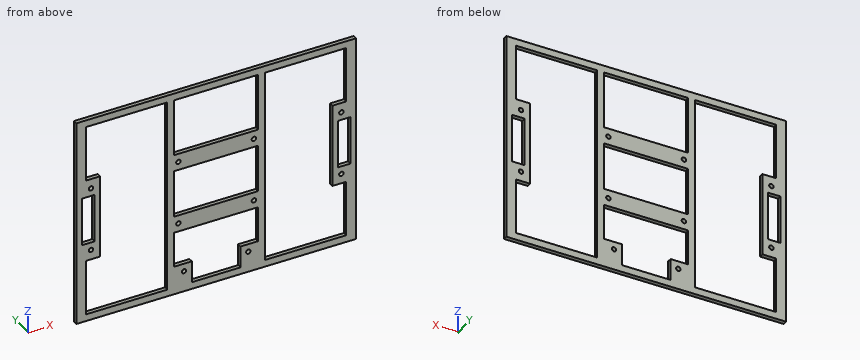
Autodesk Inventor part; units mm, degrees
ref_plane "YZ Plane" through (0, 0, 0) normal (1, 0, 0) x (0, 1, 0)
ref_plane "XZ Plane" through (0, 0, 0) normal (0, 1, 0) x (-1, 0, 0)
ref_plane "XY Plane" through (0, 0, 0) normal (0, 0, 1) x (1, 0, 0)
sketch "Skizze1" plane through (0, 0, 0) normal (0, 1, 0) x (-1, 0, 0)
  line L0 (100, -75) -> (-100, -75)
  line L1 (-100, -75) -> (-100, 75)
  line L2 (-100, 75) -> (100, 75)
  line L3 (100, 75) -> (100, -75)
  line L4 (0, -105) -> (0, 105)
  line L5 (-140, 0) -> (140, 0)
  point P0 (0, 0)
  dimension "d0" = 200
  dimension "d1" = 150
extrude "Extrusion1" add sketch "Skizze1" along normal blind 3
sketch "Skizze11" plane through (0, 3, 0) normal (0, 1, 0) x (1, 0, 0)
  circle A0 centre (27, -23) radius 1.6
  circle A1 centre (27, 23) radius 1.6
  line L0 (140, 0) -> (-140, 0)
  line L1 (100, -75) -> (100, 75)
  line L2 (100, -75) -> (100, 75)
  line L3 (0, 105) -> (0, -105)
  circle A2 centre (-27, -23) radius 1.6
  circle A3 centre (-27, 23) radius 1.6
  circle A4 centre (27, 23) radius 1.6
  circle A5 centre (-27, 23) radius 1.6
  line L4 (100, 75) -> (-100, 75)
  circle A6 centre (89.5, -23) radius 1.6
  circle A7 centre (89.5, 23) radius 1.6
  circle A8 centre (-89.5, -23) radius 1.6
  circle A9 centre (-89.5, 23) radius 1.6
  line L5 (-100, 75) -> (-100, -75)
  point P0 (0, 0)
  dimension "d50" = 3.2
  dimension "d51" = 3.2
  dimension "d52" = 23
  dimension "d53" = 23
  dimension "d54" = 73
  dimension "d55" = 73
  dimension "d62" = 3.2
  dimension "d63" = 3.2
  dimension "d64" = 27
  dimension "d65" = 27
  dimension "d66" = 52
  dimension "d67" = 52
  dimension "d70" = 3.2
  dimension "d71" = 3.2
  dimension "d72" = 23
  dimension "d73" = 23
  dimension "d74" = 10.5
  dimension "d75" = 10.5
  dimension "d76" = 3.2
  dimension "d77" = 3.2
  dimension "d78" = 10.5
  dimension "d79" = 10.5
  dimension "d80" = 23
  dimension "d81" = 23
extrude "Extrusion12" cut sketch "Skizze11" against normal up to surface (3 mm away) contours A0 | A1
extrude "Extrusion13" cut sketch "Skizze11" against normal up to surface (3 mm away) contours A2 | A3
extrude "Extrusion14" cut sketch "Skizze11" against normal up to surface (3 mm away) contours A1 | A3
extrude "Extrusion15" cut sketch "Skizze11" against normal up to surface (3 mm away) contours A6 | A7 | A8 | A9
sketch "Skizze12" plane through (0, 3, 0) normal (0, 1, 0) x (1, 0, 0)
  circle A0 centre (-23, 60) radius 1.6
  circle A1 centre (23, 60) radius 1.6
  line L0 (0, 105) -> (0, -105)
  line L1 (100, 75) -> (-100, 75)
  point P0 (0, 0)
  dimension "d84" = 3.2
  dimension "d85" = 3.2
  dimension "d86" = 23
  dimension "d87" = 23
  dimension "d88" = 15
  dimension "d89" = 15
extrude "Extrusion16" cut sketch "Skizze12" against normal up to surface (3 mm away)
sketch "Skizze13" plane through (0, 3, 0) normal (0, 1, 0) x (1, 0, 0)
  line L0 (-93, -70) -> (-35, -70)
  line L1 (-35, -70) -> (-35, 70)
  line L2 (-35, 70) -> (-93, 70)
  line L3 (35, -70) -> (93, -70)
  line L4 (93, 70) -> (35, 70)
  line L5 (35, 70) -> (35, -70)
  line L6 (-100, -75) -> (100, -75)
  line L7 (-100, 75) -> (-100, -75)
  line L8 (100, 75) -> (-100, 75)
  line L9 (100, -75) -> (100, 75)
  line L10 (-30, -70) -> (30, -70)
  line L11 (35, -70) -> (35, -30)
  line L12 (30, -29) -> (-30, -29)
  line L13 (-35, -30) -> (-35, -70)
  line L14 (-30, 29) -> (30, 29)
  line L15 (35, 29) -> (35, 54)
  line L16 (-35, 54) -> (-35, 29)
  line L17 (-30, -70) -> (-30, -29)
  line L18 (30, -70) -> (30, -29)
  line L19 (-30, 29) -> (-30, 54.4)
  line L20 (30, 29) -> (30, 54.4)
  line L21 (-93, 30) -> (-83, 30)
  line L22 (-83, 30) -> (-83, -30)
  line L23 (-83, -30) -> (-93, -30)
  line L24 (140, 0) -> (-140, 0)
  line L25 (-93, 70) -> (-93, 30)
  line L26 (-93, -30) -> (-93, -70)
  line L27 (93, 30) -> (83, 30)
  line L28 (83, 30) -> (83, -30)
  line L29 (83, -30) -> (93, -30)
  line L30 (93, -70) -> (93, -30)
  line L31 (93, 30) -> (93, 70)
  line L32 (-30, 17) -> (30, 17)
  line L33 (30, 17) -> (30, -17)
  line L34 (30, -17) -> (-30, -17)
  line L35 (-30, -17) -> (-30, 17)
  line L36 (-30, 17) -> (30, -17) construction
  line L37 (30, 17) -> (-30, -17) construction
  line L38 (-17.4, 70) -> (17.4, 70)
  line L39 (17.4, 70) -> (17.4, 54.4)
  line L40 (-17.4, 54.4) -> (-17.4, 70)
  line L41 (-17.4, 70) -> (17.4, 54.3035) construction
  line L42 (17.4, 70) -> (-17.4, 54.3035) construction
  line L43 (30, 54.4) -> (17.4, 54.4)
  line L44 (-17.4, 54.4) -> (-30, 54.4)
  circle A0 centre (-23, 60) radius 1.6
  circle A1 centre (23, 60) radius 1.6
  line L45 (87, 17.4) -> (96, 17.4)
  line L46 (96, 17.4) -> (96, -17.4)
  line L47 (96, -17.4) -> (87, -17.4)
  line L48 (87, -17.4) -> (87, 17.4)
  line L49 (87, 17.4) -> (96, -17.4) construction
  line L50 (96, 17.4) -> (87, -17.4) construction
  circle A2 centre (89.5, -23) radius 1.6
  line L51 (-96, 17.4) -> (-87, 17.4)
  line L52 (-87, 17.4) -> (-87, -17.4)
  line L53 (-87, -17.4) -> (-96, -17.4)
  line L54 (-96, -17.4) -> (-96, 17.4)
  line L55 (-96, 17.4) -> (-87, -17.4) construction
  line L56 (-87, 17.4) -> (-96, -17.4) construction
  circle A3 centre (-89.5, 23) radius 1.6
  point P0 (0, 0)
  point P1 (0, 62.1518)
  point P2 (91.5, 0)
  point P3 (-91.5, 0)
  dimension "d94" = 5
  dimension "d96" = 5
  dimension "d97" = 65
  dimension "d99" = 65
  dimension "d100" = 40
  dimension "d101" = 25
  dimension "d103" = 5
  dimension "d104" = 5
  dimension "d105" = 5
  dimension "d106" = 5
  dimension "d107" = 10
  dimension "d108" = 60
  dimension "d109" = 17
  dimension "d110" = 7
  dimension "d111" = 10
  dimension "d112" = 60
  dimension "d113" = 17
  dimension "d114" = 7
  dimension "d115" = 5
  dimension "d116" = 12
  dimension "d117" = 17
  dimension "d118" = 12
  dimension "d119" = 5
  dimension "d120" = 5
  dimension "d121" = 4
  dimension "d122" = 4
  dimension "d123" = 4
  dimension "d124" = 4
  dimension "d126" = 5.6
  dimension "d127" = 4
  dimension "d128" = 4
  dimension "d129" = 4
  dimension "d130" = 4
  dimension "d131" = 4
extrude "Extrusion17" cut sketch "Skizze13" against normal up to surface (3 mm away) contours L26 L23 L22 L24 L1 L0 | L24 L22 L21 L25 L2 L1 | L35 L32 L33 L24 | L24 L33 L34 L35 | L52 L53 L54 L24 | L24 L54 L51 L52 | L24 L28 L29 L30 L3 L5 | L5 L4 L31 L27 L28 L24 | L48 L45 L46 L24 | L24 L46 L47 L48 | L17 L12 L18 L10 | L19 L44 L40 L38 L39 L43 L20 L14
properties part number "_3D-Druck"
The model under review builds one solid part; all positions refer to its coordinate system, in mm. Round coordinates to 2 decimals unless told otherwise and drop trailing zeros. Write each loop counter-clockwise with the first axis right and the second up, starting at its lowest first coordinate (ties: lowest second). Pieces come first, ordered by that corner, then holes. Notation, with made-up numbers: M 51,-23.5 L 109,-23.5 A9 cw 109,-15.5 Z; hole C -14.5,-9 d1. An arc over 180 degrees is marked long. Answer as CSV lines item,"result". Start each with the question number.
Q1. Consider section A-A, the plane z = 2.5. Give the boundary of the cut face in (x, y), then the cut area to 3 significant figures.
Q2. Consider section B-B, the plane x = 48. Give the boundary of the cut face in (y, z), then the cut area to 3 significant figures.
Q3. Wall thickness on line 1 along Z through (x, y) = (89.5, 2.2); line 2 along Z through (x, y) = (12.5, 0.9); line 3 along Z through (x, y) = (-27, 1.4): over which ranges is each line inside the solid? List them lowest first.
Q4. Clearance check with a flat-ended pin moving along its axis: P1, Ø6, axis at x = -16, z = -52.5, coming from the +Y side. State where the tip first meets the part, or that it passes through.
Q5. Consider section C-C, the plane y = 1.5. State how many separate pieces and enclosed holes the cut face has, then the cut area to 3 significant figures.
Result set:
1,outline,"M -100,0 L -96,0 L -96,3 L -100,3 Z; M -87,0 L -83,0 L -83,3 L -87,3 Z; M -35,0 L -30,0 L -30,3 L -35,3 Z; M 30,0 L 35,0 L 35,3 L 30,3 Z; M 83,0 L 87,0 L 87,3 L 83,3 Z; M 96,0 L 100,0 L 100,3 L 96,3 Z"
1,area,"78.0 mm²"
2,outline,"M 0,-75 L 3,-75 L 3,-70 L 0,-70 Z; M 0,70 L 3,70 L 3,75 L 0,75 Z"
2,area,"30.0 mm²"
3,line 1,"z = -75 to -70, -30 to -24.6, -21.4 to -17.4, 17.4 to 21.4, 24.6 to 30, 70 to 75"
3,line 2,"z = -75 to -70, -29 to -17, 17 to 29, 70 to 75"
3,line 3,"z = -75 to -54.4, -29 to -24.6, -21.4 to -17, 17 to 21.4, 24.6 to 29, 70 to 75"
4,P1,"stops at y = 3"
5,separate pieces,"1"
5,enclosed holes,"17"
5,area,"7,690 mm²"
